Geometry: final body of the model. Coordinates: model frame, mm. Face numbers are marked on the shaded views. A direction names the side the tool comes from. Round coordinates to 2 decimals unless told otherwise and drop trailing zeros. Loops run counter-clockwise (first coordinate to the right, second up) from the corner with the lowest first, then second, coordinate; pieces in that order, holes last. Notation, with made-up numbers: M 70,-4 L 77,-4 A28 cw 77,21 Z; hole C 34.25,19 d8. An arc over 180 degrees is marked long. Answer as a JSON object with one key per item and string values.
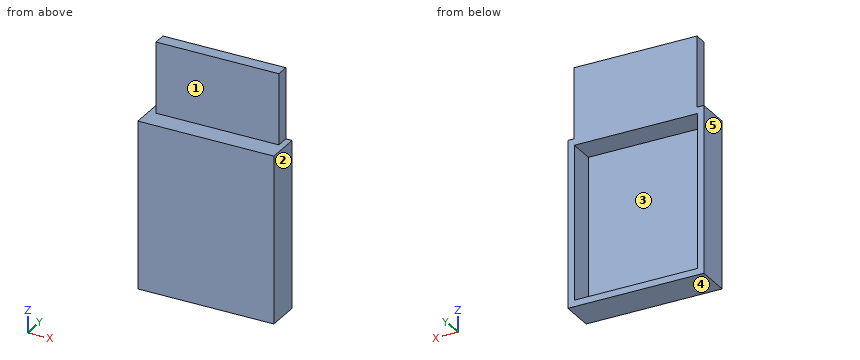
```python
from build123d import *

# Parameters (mm, degrees)
F0_W     = 134.62
F0_H     = 165.1
F0_W_2   = 121.92
F0_H_2   = 152.4
F1_DEPTH = 33.02
F2_W     = 121.92
F2_H     = 152.4
F4_DEPTH = 7.62
F5_W     = 121.666
F5_H     = 69.9852703571
F6_DEPTH = 12.7
F7_DEPTH = 5.08
F8_DEPTH = 3.81


with BuildPart() as f1:
    # F0 (on Front) → F1 (new body)
    with BuildSketch(Plane.XZ):
        with Locations((67.31, 82.55)):
            Rectangle(F0_W, F0_H)
        with Locations((67.31, 82.55)):
            Rectangle(F0_W_2, F0_H_2, mode=Mode.SUBTRACT)
    extrude(amount=F1_DEPTH)

    # F2 (on face) → F4 (join)
    with BuildSketch(Plane.XZ.offset(33.02)):
        with Locations((67.31, 82.55)):
            Rectangle(F2_W, F2_H)
    extrude(amount=-F4_DEPTH)

    # F5 (on face) → F6 (join)
    with BuildSketch(Plane(origin=(0, 0, 0), x_dir=(-1, 0, 0), z_dir=(0, 1, 0))):
        with Locations((-67.5779950066, 200.0926351786)):
            Rectangle(F5_W, F5_H)
    extrude(amount=-F6_DEPTH)

    # F7 (add): a face of the model
    f7_faces = [f1.faces().sort_by_distance(p)[0] for p in [
        (67.31, -16.51, 0),
    ]]
    extrude(f7_faces, amount=-F7_DEPTH)

    # F8 (add): a face of the model
    f8_faces = [f1.faces().sort_by_distance(p)[0] for p in [
        (67.31, -16.51, 0),
    ]]
    extrude(f8_faces, amount=-F8_DEPTH)


solid = f1.part
```
1) Line query: probe 1 along Z at (x, y) = (59, -24); probe 2 along Z at (x, y) = (72, -7.5); probe 3 along X at (y, z) = (-11.5, 68). Output: solid intervals per line, ascending.
Geometry results:
{"probe 1": "0 to 6.35, 158.75 to 165.1", "probe 2": "0 to 6.35, 158.75 to 235.09", "probe 3": "0 to 6.35, 128.27 to 134.62"}
2) Cut plane B-B on y = -17.5. Return the cut outline in (x, z), and give its area (3 significant figures).
Geometry results:
{"outline": "M 0,0 L 134.62,0 L 134.62,165.1 L 0,165.1 Z; hole M 6.35,6.35 L 128.27,6.35 L 128.27,158.75 L 6.35,158.75 Z", "area": "3,650 mm2"}
3) First-contact query: pin 1 (10 mm diameter, centred on x = 65, y = -22.5, fed in from +Z); pin 2 (10 mm diameter, centred on y = -7.5, z = 189, fed in from +X); pin 3 (14 mm diameter, centred on y = -7, z = 203.5, fed in from -X) (3 decimals). Flat tips, straight axial feed; report the tip coordinate or a pass-through.
Geometry results:
{"pin 1": "z = 165.1", "pin 2": "x = 128.41", "pin 3": "x = 6.745"}
4) Cut plane D-D on y = -29. Return the cut outline in (x, z).
Geometry results:
{"outline": "M 0,0 L 134.62,0 L 134.62,165.1 L 0,165.1 Z"}
5) Set-up query: the marked faces 1 and 2. Return all of +Z, -Z, +X, -X, +Y, -Y with unobstructed straight access to the full face (end or side cutting, diameter ignored); none if empty.
Geometry results:
{"face 1": "+Z, +X, -X, -Y", "face 2": "+Z, -Z, +X, +Y, -Y"}
6) Cut plane A-A on x = 65. Return the cut outline in (y, z).
Geometry results:
{"outline": "M -33.02,0 L 0,0 L 0,6.35 L -25.4,6.35 L -25.4,158.75 L 0,158.75 L 0,235.09 L -12.7,235.09 L -12.7,165.1 L -33.02,165.1 Z"}
7) Cut plane C-C on z = 86.5. Return the cut outline in (x, y), and give its area (3 significant figures).
Geometry results:
{"outline": "M 0,-33.02 L 134.62,-33.02 L 134.62,0 L 128.27,0 L 128.27,-25.4 L 6.35,-25.4 L 6.35,0 L 0,0 Z", "area": "1,350 mm2"}
8) Pull-direction query (X, two-part tool) for the marked faces 3, 4 and 5; classes: +X half, -X half, draft (parallel to the pull), parting line (faces both ways), or undercut.
Geometry results:
{"face 3": "undercut", "face 4": "draft", "face 5": "-X half"}
